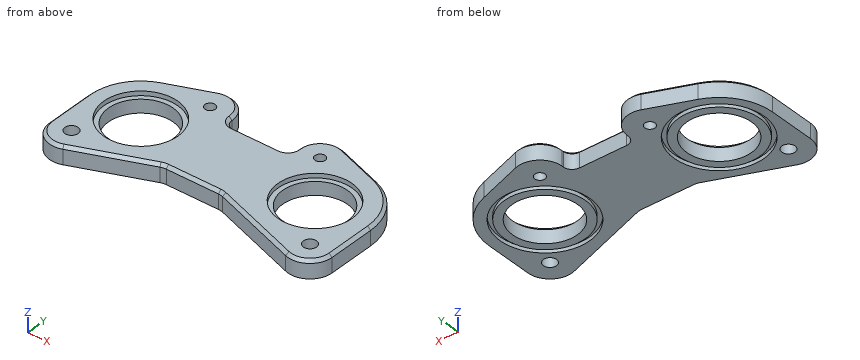
from build123d import *

# Parameters (mm, degrees)
F0_R     = 4.5
F0_R_2   = 22
F0_R_3   = 3.5
F1_DEPTH = 12
F2_R     = 25.2
F3_DEPTH = 3
F4_SIZE  = 2
F5_R     = 30.5
F5_R_2   = 27.5
F6_DEPTH = 2.5


# Not quite as in the source:
# - ends of sketch curves that miss each other by under 0.0002 mm in the source are joined


with BuildPart() as f1:
    # F0 (on Top) → F1 (new body)
    with BuildSketch(Plane.XY):
        with BuildLine():
            Line((-96.25, -7.835472), (-96.25, -39.300472))
            ThreePointArc((-96.25, -39.300472), (-89.6603385796, -51.720866719), (-75.6811726698, -53.2284353172))
            Line((-75.6811726698, -53.2284353172), (-25.901923657, -33.3251628629))
            ThreePointArc((-25.901923657, -33.3251628629), (-24.0797305928, -32.7907701516), (-22.189372, -32.610472))
            Line((-22.189372, -32.610472), (13.41096, -32.610472))
            ThreePointArc((13.41096, -32.610472), (15.0445629213, -32.7448072228), (16.6342757601, -33.1442037009))
            Line((16.6342757601, -33.1442037009), (76.4150264593, -53.4998741564))
            ThreePointArc((76.4150264593, -53.4998741564), (89.9814201421, -51.4972872524), (96.25, -39.300472))
            Line((96.25, -39.300472), (96.25, -7.385472))
            ThreePointArc((96.25, -7.385472), (89.1771507076, 14.6451910108), (70.602136617, 28.4417181588))
            Line((70.602136617, 28.4417181588), (40.3905414757, 38.7289301785))
            ThreePointArc((40.3905414757, 38.7289301785), (26.82414783, 36.7263432324), (20.555568, 24.529528))
            Line((20.555568, 24.529528), (20.555568, 23.389528))
            ThreePointArc((20.555568, 23.389528), (18.7982086871, 19.1468873129), (14.555568, 17.389528))
            Line((14.555568, 17.389528), (-17.637618, 17.389528))
            ThreePointArc((-17.637618, 17.389528), (-21.8802586871, 19.1468873129), (-23.637618, 23.389528))
            Line((-23.637618, 23.389528), (-23.637618, 23.629528))
            ThreePointArc((-23.637618, 23.629528), (-30.2272793638, 36.0499226807), (-44.2064452032, 37.557491368))
            Line((-44.2064452032, 37.557491368), (-73.4226694122, 25.875948235))
            ThreePointArc((-73.4226694122, 25.875948235), (-90.0062904382, 12.5210187268), (-96.25, -7.835472))
        make_face()
        with Locations((-81.25, -39.300472)):
            Circle(F0_R, mode=Mode.SUBTRACT)
        with Locations((-59.943809, -7.835472)):
            Circle(F0_R_2, mode=Mode.SUBTRACT)
        with Locations((81.25, -39.300472)):
            Circle(F0_R, mode=Mode.SUBTRACT)
        with Locations((-38.637618, 23.629528)):
            Circle(F0_R_3, mode=Mode.SUBTRACT)
        with Locations((58.402784, -7.385472)):
            Circle(F0_R_2, mode=Mode.SUBTRACT)
        with Locations((35.555568, 24.529528)):
            Circle(F0_R_3, mode=Mode.SUBTRACT)
    extrude(amount=F1_DEPTH)

    # F2 (on face) → F3 (cut)
    with BuildSketch(Plane.XY.offset(12)):
        with Locations((-59.943809, -7.835472)):
            Circle(F2_R)
        with Locations((58.402784, -7.385472)):
            Circle(F2_R)
    extrude(amount=-F3_DEPTH, mode=Mode.SUBTRACT)

    # F4
    f4_edges = [f1.edges().sort_by_distance(p)[0] for p in [
        (-58.814557, 31.71672, 12),
    ]]
    chamfer(f4_edges, length=F4_SIZE)

    # F5 (on face) → F6 (cut)
    with BuildSketch(Plane(origin=(0, 0, 0), x_dir=(1, 0, 0), z_dir=(0, 0, -1))):
        with Locations((-59.943809, 7.835472)):
            Circle(F5_R)
        with Locations((-59.943809, 7.835472)):
            Circle(F5_R_2, mode=Mode.SUBTRACT)
        with Locations((58.402784, 7.385472)):
            Circle(F5_R)
        with Locations((58.402784, 7.385472)):
            Circle(F5_R_2, mode=Mode.SUBTRACT)
    extrude(amount=-F6_DEPTH, mode=Mode.SUBTRACT)


solid = f1.part
The listing builds one solid part. Answer for the finished solid, in the listing's coordinates (mm). Coordinates: 2 decimals unless noted, no trailing zeros. Order: outer loops, then holes, each group sorted by start corner. A loop starts at its lowest first (then second) coordinate and runs counter-clockwise, first axis right, second up.
Q1. A cutting plane is placed at C-C, the plane y = 5. State how many separate pieces and enclosed holes the cut face has, and give its area (3 significant figures).
Q2. A cutting plane is placed at A-A, the plane z = 5.75. Write down the section's boundary in (x, y).
Q3. Given P1, Ø0.9, axis at y = 24, z = 5, coming from the -X side; P2, Ø11.5, axis at x = 81.25, y = -39.3, coming from the +Z side; P3, Ø4, axis at x = -60, z = 2, coming from the -Y side; P4, Ø5, axis at x = 4.5, z = 5, coming from the +Y side, each flat-ended and moving along its own axis, determine where each tip first touches the part or whether it passes through.
Q4. A cutting plane is placed at B-B, the plane x = 49. Write down the section's boundary in (y, z).
Q5. Consider line 1 (X direction, y = -15, z = 4); line 2 (X direction, y = 25, z = 6.5); line 3 (X direction, y = -26, z = 4.5). Determine where each line is inside the solid, lowest interval first.
Answers follow:
1. separate pieces: 3
1. enclosed holes: 0
1. area: 1,310 mm2
2. outline: (-96.25, -39.3) arc R15 ccw to (-75.68, -53.23) - (-25.9, -33.33) arc R10 cw to (-22.19, -32.61) - (13.41, -32.61) arc R10 cw to (16.63, -33.14) - (76.42, -53.5) arc R15 ccw to (96.25, -39.3) - (96.25, -7.39) arc R37.85 ccw to (70.6, 28.44) - (40.39, 38.73) arc R15 ccw to (20.56, 24.53) - (20.56, 23.39) arc R6 cw to (14.56, 17.39) - (-17.64, 17.39) arc R6 cw to (-23.64, 23.39) - (-23.64, 23.63) arc R15 ccw to (-44.21, 37.56) - (-73.42, 25.88) arc R36.31 ccw to (-96.25, -7.84) - close; hole circle Ø9 at (-81.25, -39.3); hole circle Ø44 at (-59.94, -7.84); hole circle Ø7 at (-38.64, 23.63); hole circle Ø7 at (35.56, 24.53); hole circle Ø44 at (58.4, -7.39); hole circle Ø9 at (81.25, -39.3)
3. P1: stops at x = -78.19
3. P2: stops at z = 12
3. P3: stops at y = -47.76
3. P4: stops at y = 17.39
4. outline: (-44.16, 0) - (-36.4, 0) - (-36.4, 2.5) - (-33.23, 2.5) - (-33.23, 0) - (-27.27, 0) - (-27.27, 9) - (-30.77, 9) - (-30.77, 12) - (-42.05, 12) - (-44.16, 10) - close; (12.5, 0) - (18.46, 0) - (18.46, 2.5) - (21.63, 2.5) - (21.63, 0) - (35.8, 0) - (35.8, 10) - (33.68, 12) - (15.99, 12) - (15.99, 9) - (12.5, 9) - close
5. line 1: x = -96.25 to -80.74, -39.14 to 37.76, 79.04 to 96.25
5. line 2: x = -75.43 to -41.86, -35.42 to -23.7, 20.56 to 32.09, 39.02 to 77.99
5. line 3: x = -96.25 to -72.36, -47.53 to 46.68, 70.13 to 96.25
